Here's the drawing with two shaded views (mm, measured from the low corner). I have some questions. A direction names the side the tool comes from. Coordinates: 2 decimals unless noted, no trailing zeros. Write each loop counter-clockwise with the first axis right and the second up, starting at its lowest first coordinate (ties: lowest second). Pieces come first, ordered by that corner, then holes. Notation, with made-up numbers: (15, 86.25) -> (49, 86.25) arc R18 cw to (49, 99.25) -> close; hole circle Ø11 at (-10.5, 49). An arc over 180 degrees is marked (long way). Put each result on its own line as item: value.
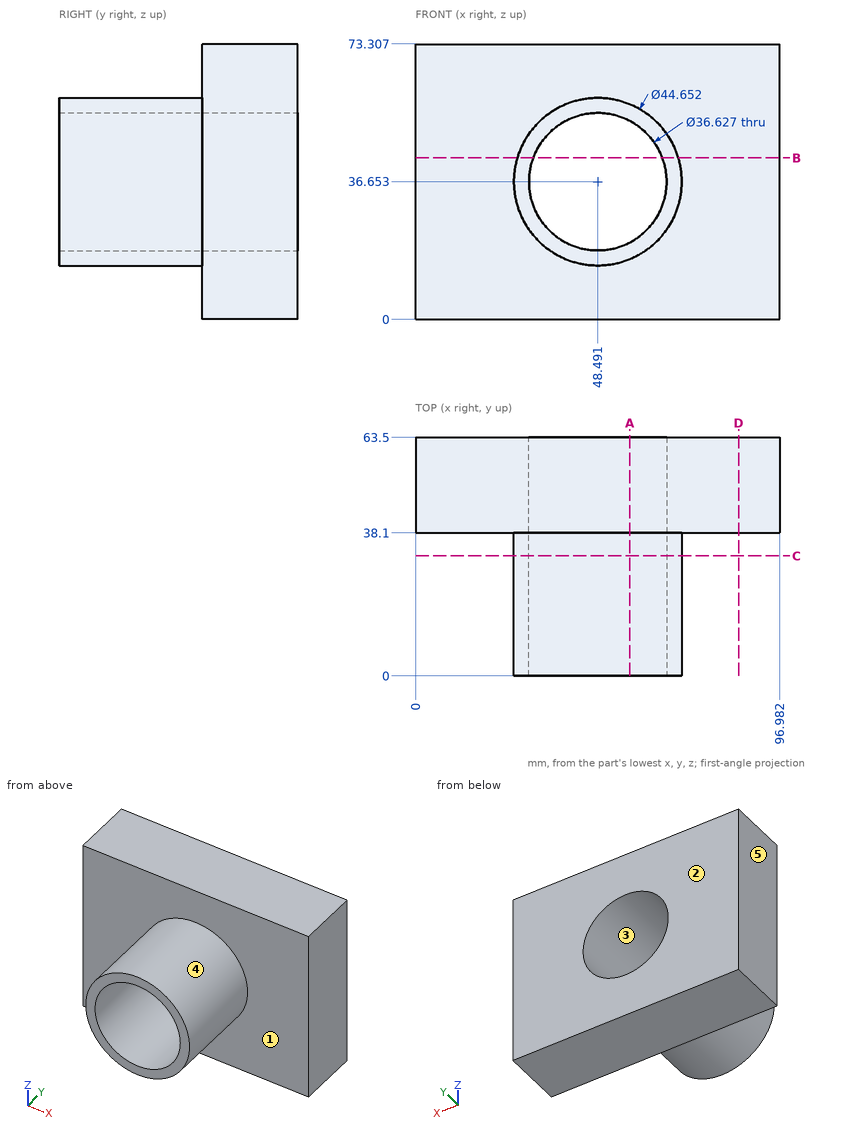
Item 1: Imagine slicing it at D-D on x = 86. Write out the boundary of the cut face in (y, z).
Output:
outline: (38.1, 0) -> (63.5, 0) -> (63.5, 73.31) -> (38.1, 73.31) -> close
Item 2: Imagine slicing it at A-A on x = 57. Write out the boundary of the cut face in (y, z) (1 decimal).
Output:
outline: (0, 16) -> (38.1, 16) -> (38.1, 0) -> (63.5, 0) -> (63.5, 20.4) -> (0, 20.4) -> close; (0, 52.9) -> (63.5, 52.9) -> (63.5, 73.3) -> (38.1, 73.3) -> (38.1, 57.3) -> (0, 57.3) -> close
Item 3: For P1, Ø8, axis at y = 18.5, z = 45, coming from the -X side; P2, Ø10, axis at x = 42, z = 65, coming from the -Y side; P3, Ø6, axis at x = 37.5, z = 30, coming from the -Y side, each with a flat end and sliding along its axis, tell me the tip position at first contact or that it passes through.
Output:
P1: stops at x = 26.59
P2: stops at y = 38.1
P3: passes through
Item 4: Please list where these lines run through material, in increasing order: line 1 along Y through (x, z) = (80, 12); line 2 along Z through (x, y) = (64, 58) (1 decimal); line 3 along Z through (x, y) = (65, 53) (1 decimal). Write a range as from..to.
Output:
line 1: y = 38.1..63.5
line 2: z = 0..26.9, 46.4..73.3
line 3: z = 0..28.7, 44.6..73.3
Item 5: Imagine slicing it at C-C on y = 32. Write out the boundary of the cut face in (x, z) (1 decimal).
Output:
outline: circle Ø44.7 at (48.5, 36.7); hole circle Ø36.6 at (48.5, 36.7)
Item 6: Which directions (+Z, -Z, +X, -X, +Y, -Y) give clear straight access to the entire face, cutting with the end or side of a thin tool? Please do the marked faces 1 and 2.
Output:
face 1: -Y
face 2: +Z, -Z, +X, -X, +Y
Item 7: Imagine slicing it at B-B on z = 43. Write out the boundary of the cut face in (x, y) (1 decimal), then the cut area to 3 significant figures.
Output:
outline: (0, 38.1) -> (27.1, 38.1) -> (27.1, 0) -> (31.3, 0) -> (31.3, 63.5) -> (0, 63.5) -> close; (65.7, 0) -> (69.9, 0) -> (69.9, 38.1) -> (97, 38.1) -> (97, 63.5) -> (65.7, 63.5) -> close
area: 1,910 mm²
Item 8: If we mould it in two halves opening along Z, with no side actions, what happens to the marked faces 3, 4 and 5? For each: released by +Z, released by -Z, zero draft, split by the parting line, or undercut.
Output:
face 3: undercut
face 4: split by the parting line
face 5: zero draft
